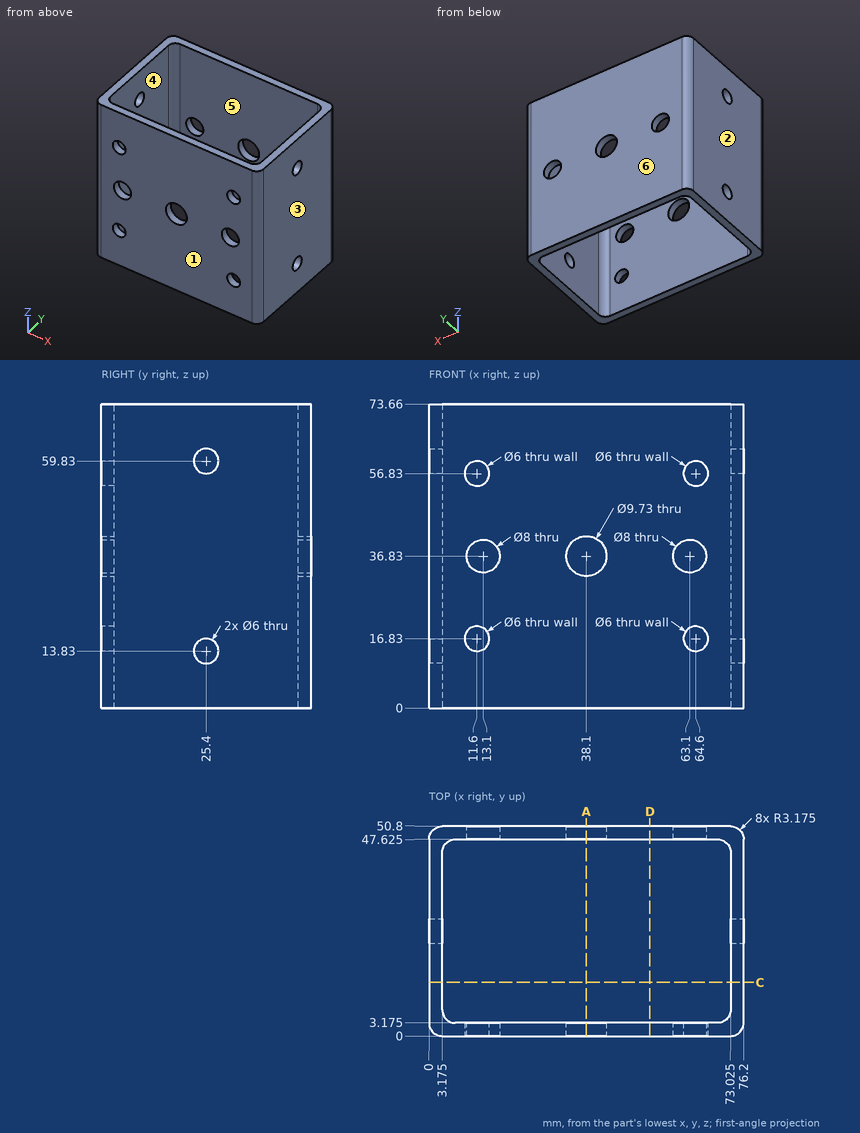
Input: dimensioned drawing with shaded views. Units: mm. Origin: part minimum x, y, z. A direction names the side the tool comes from. Round coordinates to 2 decimals unless told otherwise and drop trailing zeros. Loops run counter-clockwise (first coordinate to the right, second up) from the corner with the lowest first, then second, coordinate; pieces in that order, holes last. Notation, with made-up numbers: (24.25, 74.5) -> (82.25, 74.5) arc R14 cw to (82.25, 85.5) -> close; hole circle Ø4 at (-12, 27). An arc over 180 degrees is marked (long way). Answer as a JSON object with one key per item and string values. Group by question number.
Q1. Access query for the marked faces 5 and 6. Directions: +Z, -Z, +X, -X, +Y, -Y. A direction counts if a zero-diameter tool reaches every point of the face in a straight line with its end or side. Return the directions, or none.
Q2. Ray query, line 1 (X direction, y = 34, z = 28) (1 decimal); line 2 (Y direction, x = 43.5, z = 26) (1 decimal); line 3 (Z direction, x = 2, y = 25). Return the intervals inside material, ascending. Write a range as from..to.
Q3. Mould query, pull axis X, two halves, no side actions, for the marked faces 1, 2, 3 and 4. Classes: pulls with the +X half, pulls with the -X half, needs draft (parallel to the pull), parting line crosses it, or undercut.
Q4. Section query C-C (y = 13). Output: boundary loops of the cut face in (x, z) (1 decimal).
Q5. Section query A-A (x = 38.1). Output: boundary loops of the cut face in (y, z) (1 decimal), plus the area to 3 significant figures.
Q6. Section query D-D (x = 53.5). Output: boundary loops of the cut face in (y, z) (1 decimal).
Completed:
{
 "1": {"face 5": "+Z, -Z", "face 6": "+Z, -Z, +X, -X, +Y"},
 "2": {"line 1": "0..3.2, 73..76.2", "line 2": "0..3.2, 47.6..50.8", "line 3": "0..10.86, 16.8..56.86, 62.8..73.66"},
 "3": {"face 1": "needs draft", "face 2": "pulls with the -X half", "face 3": "pulls with the +X half", "face 4": "undercut"},
 "4": {"outline": "(0, 0) -> (3.2, 0) -> (3.2, 73.7) -> (0, 73.7) -> close; (73, 0) -> (76.2, 0) -> (76.2, 73.7) -> (73, 73.7) -> close"},
 "5": {"outline": "(0, 0) -> (3.2, 0) -> (3.2, 32) -> (0, 32) -> close; (0, 41.7) -> (3.2, 41.7) -> (3.2, 73.7) -> (0, 73.7) -> close; (47.6, 0) -> (50.8, 0) -> (50.8, 32) -> (47.6, 32) -> close; (47.6, 41.7) -> (50.8, 41.7) -> (50.8, 73.7) -> (47.6, 73.7) -> close", "area": "406 mm²"},
 "6": {"outline": "(0, 0) -> (3.2, 0) -> (3.2, 73.7) -> (0, 73.7) -> close; (47.6, 0) -> (50.8, 0) -> (50.8, 73.7) -> (47.6, 73.7) -> close"}
}
